Geometry check sheet. Reference: drawing and pictorial views, mm from the part's lowest x, y, z. A direction names the side the tool comes from. Give positions to 0.01 mm unless a question says otherwise; leave off trailing zeros. Write each loop counter-clockwise with the first axis right and the second up, starting at its lowest first coordinate (ties: lowest second). Pieces come first, ordered by that corner, then holes. Notation, with made-up numbers: M 29.25,-7 L 78.25,-7 A22 ccw 78.25,21 Z; hole C -11.75,-32.75 d9. An arc over 180 degrees is marked long. Answer as a JSON object with one key per item and string values.
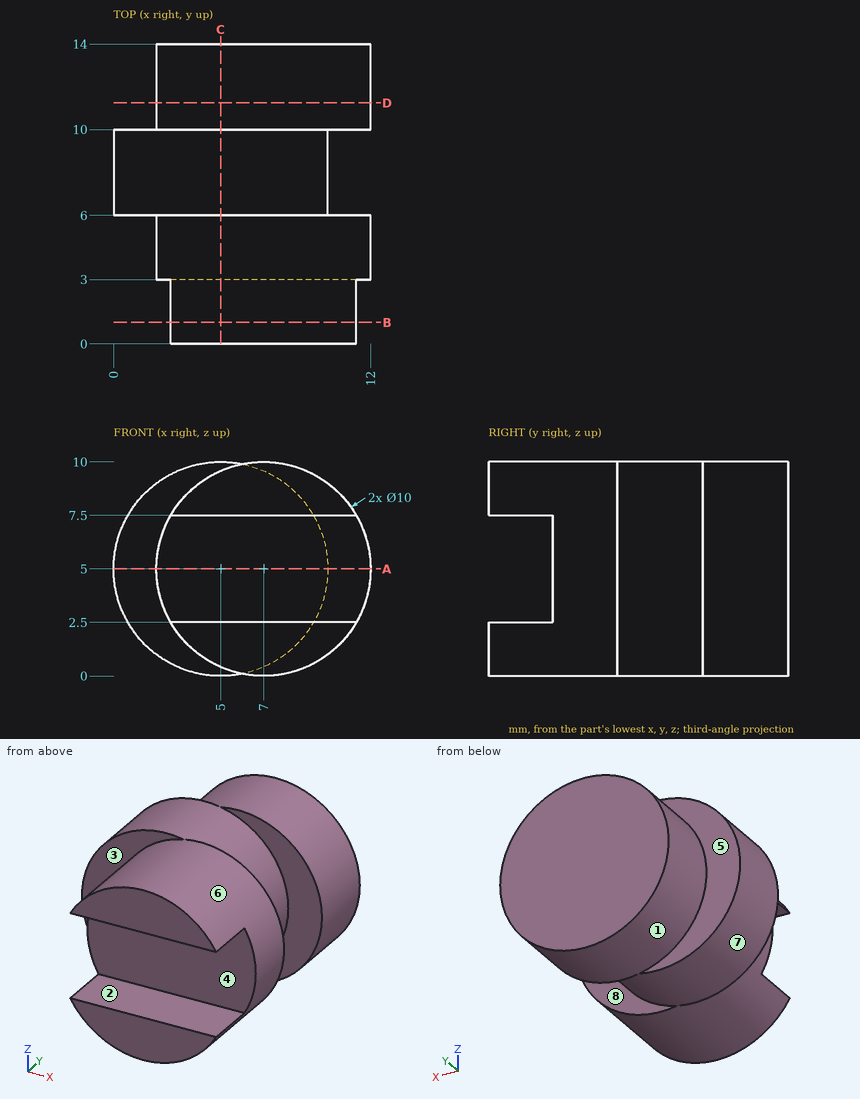
1) Section check A-A on z = 5. Record the boundary of the cut face in (x, y), and give its area (3 significant figures).
Completed:
{"outline": "M 0,6 L 2,6 L 2,3 L 12,3 L 12,6 L 10,6 L 10,10 L 12,10 L 12,14 L 2,14 L 2,10 L 0,10 Z", "area": "110 mm2"}
2) Thickness scan on L1, parallel to Y at x = 10, z = 3.25; L2, parallel to X at y = 13.25, z = 7.5; L3, parallel to Y at x = 1.5, z = 8.25. Record the ranges inside material, lowest first.
Completed:
{"L1": "y = 3 to 6, 10 to 14", "L2": "x = 2.67 to 11.33", "L3": "y = 6 to 10"}
3) Go/stop test with flat-tipped pins: pin 1 (3 mm diameter, centred on y = 3.5, z = 3, fed in from +X); pin 2 (1 mm diameter, centred on x = 2, z = 5, fed in from -Y); pin 3 (4 mm diameter, centred on x = 2.5, y = 3, fed in from +Z). Record where each tip stops, or that it passes through.
Completed:
{"pin 1": "stops at x = 11.97", "pin 2": "stops at y = 3", "pin 3": "stops at z = 9.33"}
4) Section check D-D on y = 11.25. Record the boundary of the cut face in (x, z).
Completed:
{"outline": "C 7,5 d10"}
5) Section check B-B on y = 1. Record the boundary of the cut face in (x, z), and give its area (3 significant figures).
Completed:
{"outline": "M 2.67,2.5 A5 ccw 11.33,2.5 Z; M 2.67,7.5 L 11.33,7.5 A5 ccw Z", "area": "30.7 mm2"}
6) Release check for a two-part mould opening along Z. For the marked faces 1, 2 and 3 record: pulls with the +Z half, pulls with the -Z half, needs draft (parallel to the pull), parting line crosses it, or undercut.
Completed:
{"face 1": "parting line crosses it", "face 2": "undercut", "face 3": "needs draft"}
7) Access from +Z, -Z, +X, -X, +Y, -Y to the whole of each face (thin tool, end or side, straight path). Record for the marked faces 4, 5, 6, 7 and 8.
Completed:
{"face 4": "+X, -X, -Y", "face 5": "-X, +Y", "face 6": "-Y", "face 7": "none", "face 8": "+X"}
8) Section check C-C on x = 5. Record the boundary of the cut face in (y, z).
Completed:
{"outline": "M 0,0.42 L 6,0.42 L 6,0 L 10,0 L 10,0.42 L 14,0.42 L 14,9.58 L 10,9.58 L 10,10 L 6,10 L 6,9.58 L 0,9.58 L 0,7.5 L 3,7.5 L 3,2.5 L 0,2.5 Z"}
